Design review of the part built by this model. Coordinates are the model's own, in mm. A direction names the side the tool comes from. Round coordinates to 2 decimals unless told otherwise and drop trailing zeros. Write each loop counter-clockwise with the first axis right and the second up, starting at its lowest first coordinate (ties: lowest second). Pieces come first, ordered by that corner, then holes. Notation, with made-up numbers: (73.25, 5.25) -> (132.25, 5.25) arc R17 ccw to (132.25, 27.25) -> close; hole circle Ø5 at (-10.75, -10). An arc over 180 degrees is marked (long way). One line per question, with ' | ' between items. Start each with the question number.
1) Mouldability with a two-part tool opening along X and no side actions: class faces 5 (the cylindrical face through (-2.17, 13.85, 17.91)), 6 (the cylindrical face through (-13.434, 12.862, 16.727)), 7 (the flat face through (-12, 3, 19)) as +X half, -X half, draft (parallel to the pull), parting line (faces both ways), or undercut.
2) Consider section D-D (y = 3.2). Give the boundary of the cut face in (x, z).
3) Consider section A-A (y = 14.7). Give the boundary of the cut face in (x, z), then the cut area to 3 significant figures.
4) For faces 1 (the flat face through (-3, 6, 19)), 2 (the flat face through (-11, 10, 11.6)), 3 (the flat face through (-9, 21, 17)), 4 (the flat face through (-15, 6, 19)), list the 3-axis set-ups (+Z, -Z, +X, -X, +Y, -Y) from which the entire face can be reached by the end or side of a thin tool; tool diameter is ignored.
5) Consider section B-B (x = -9). Give the boundary of the cut face in (y, z).
6) Consider section C-C (z = 5.25). Give the boundary of the cut face in (x, y), then the cut area to 3 significant figures.
7) Insertion check: pin 1 Ø2 at (x, y) = (-15, 13) entering from -Z; pin 2 Ø9.5 at (x, z) = (-11, 4.5) entering from +Y; pin 3 Ø4 at (x, y) = (-3.25, 3.2) entering from +Z; pin 4 Ø6 at (x, z) = (-12.5, 9) entering from -Y. Each pin has a flat end and moves straight along its axis. Give the tip position at first contact, or say it passes through.
8) For probe 1 along Y at (x, z) = (-14.75, 11.25); probe 2 along Y at (x, z) = (-9, 17.5); probe 3 along Y at (x, z) = (-6.5, 10.75), list the stretches that pass through material, from the lowest coordinate up.
Autodesk Inventor part; units mm, degrees
ref_plane "YZ Plane" through (0, 0, 0) normal (1, 0, 0) x (0, 1, 0)
ref_plane "XZ Plane" through (0, 0, 0) normal (0, 1, 0) x (-1, 0, 0)
ref_plane "XY Plane" through (0, 0, 0) normal (0, 0, 1) x (1, 0, 0)
sketch "Sketch1" plane through (0, 0, 0) normal (0, 0, 1) x (1, 0, 0)
  line L0 (0, 0) -> (-18, 0)
  line L1 (-18, 0) -> (-18, 6)
  line L2 (-18, 6) -> (0, 6)
  line L3 (0, 6) -> (0, 0)
  dimension "d0" = 18
  dimension "d1" = 6
extrude "Extrusion1" add sketch "Sketch1" along normal blind 22
sketch "Sketch2" plane through (0, 0, 22) normal (0, 0, 1) x (1, 0, 0)
  line L0 (-18, 0) -> (0, 0)
  line L1 (0, 0) -> (0, 6)
  line L2 (0, 6) -> (-18, 6)
  line L3 (-18, 6) -> (-18, 0)
  circle A0 centre (-14.75, 3.2) radius 1.25
  circle A1 centre (-3.25, 3.2) radius 1.25
  dimension "d4" = 2.5
  dimension "d5" = 2.5
  dimension "d6" = 2.8
  dimension "d7" = 2.8
  dimension "d8" = 3.25
  dimension "d9" = 3.25
  dimension "d31" = 11.5
extrude "Extrusion2" cut sketch "Sketch2" against normal through all contours A0 | A1
sketch "Sketch3" plane through (0, 0, 0) normal (1, 0, 0) x (0, 0, -1)
  line L0 (0, 6) -> (0, 0)
  line L1 (0, 6) -> (-22, 6)
  line L2 (-22, 0) -> (-22, 6)
  line L3 (0, 0) -> (-22, 0)
  line L4 (0, 6) -> (-22, 6)
  line L5 (-22, 6) -> (-11.6, 6)
  line L6 (-11.6, 6) -> (-11.6, 21)
  line L7 (-11.6, 21) -> (-22, 21)
  line L8 (-22, 21) -> (-22, 6)
  dimension "d12" = 10.4
  dimension "d13" = 15
extrude "Extrusion3" add sketch "Sketch3" against normal up to surface (18 mm away) contours L1 L8 L7 L6
sketch "Sketch4" plane through (0, 6, 11.6) normal (0, 0, -1) x (-1, 0, 0)
  line L0 (18, 0) -> (18, 15)
  line L1 (0, 15) -> (18, 15)
  line L2 (0, 15) -> (0, 0)
  line L3 (18, 0) -> (0, 0)
  circle A0 centre (9, 8.7) radius 4.8
  point P0 (0, -6)
  dimension "d16" = 9.6
  dimension "d17" = 6.3
extrude "Extrusion4" cut sketch "Sketch4" against normal through all contours A0
sketch "Sketch5" plane through (-18, 0, 0) normal (-1, 0, 0) x (0, 0, 1)
  line L0 (22.0213, 0) -> (16.0213, 0)
  line L1 (16.0213, 0) -> (16.0213, 6)
  line L2 (16.0213, 6) -> (22.0213, 6)
  line L3 (22.0213, 6) -> (22.0213, 0)
  point P0 (0, 0)
  dimension "d20" = 6
  dimension "d21" = 6
extrude "Extrusion5" cut sketch "Sketch5" against normal blind 6
sketch "Sketch6" plane through (0, 0, 0) normal (1, 0, 0) x (0, 0, -1)
  line L0 (-22, 6) -> (-22, 0)
  line L1 (-16.0213, 6) -> (-22, 6)
  line L2 (-16.0213, 0) -> (-16.0213, 6)
  line L3 (-22, 0) -> (-16.0213, 0)
  point P0 (0, 0)
extrude "Extrusion6" cut sketch "Sketch6" against normal blind 6
sketch "Sketch7" plane through (0, 0, 0) normal (1, 0, 0) x (0, 0, -1)
  line L0 (-6.6, 12.2) -> (-11.6, 12.2)
  line L1 (-6.6, 17.2) -> (-11.6, 17.2)
  line L2 (-11.6, 21) -> (-11.6, 6)
  line L3 (-22, 6) -> (-22, 21)
  circle A0 centre (-16.8, 14.7) radius 1.4
  point P0 (0, 0)
  dimension "d26" = 2.8
  dimension "d27" = 5.2
  dimension "d28" = 2.5
extrude "Extrusion7" cut sketch "Sketch7" against normal blind 6
equation "\"d9\" = d8"
properties part number "00_micrometer_moun_xystage_china_new"
From the geometry:
1) face 5: draft | face 6: undercut | face 7: -X half
2) outline: (-18, 0) -> (-16, 0) -> (-16, 16.02) -> (-18, 16.02) -> close; (-13.5, 0) -> (-4.5, 0) -> (-4.5, 16.02) -> (-6, 16.02) -> (-6, 22) -> (-12, 22) -> (-12, 16.02) -> (-13.5, 16.02) -> close; (-2, 0) -> (0, 0) -> (0, 16.02) -> (-2, 16.02) -> close
3) outline: (-18, 11.6) -> (-13.8, 11.6) -> (-13.8, 22) -> (-18, 22) -> close; (-4.2, 11.6) -> (0, 11.6) -> (0, 15.4) -> (-4.2, 15.4) -> close; (-4.2, 18.2) -> (0, 18.2) -> (0, 22) -> (-4.2, 22) -> close | area: 75.6 mm2
4) face 1: +Z, +X, -Y | face 2: -Z, +X, -X, +Y | face 3: +Z, -Z, +X, -X, +Y | face 4: +Z, -X, -Y
5) outline: (0, 0) -> (6, 0) -> (6, 11.6) -> (9.9, 11.6) -> (9.9, 22) -> (0, 22) -> close; (19.5, 11.6) -> (21, 11.6) -> (21, 22) -> (19.5, 22) -> close
6) outline: (-18, 0) -> (0, 0) -> (0, 6) -> (-18, 6) -> close; hole circle Ø2.5 at (-14.75, 3.2); hole circle Ø2.5 at (-3.25, 3.2) | area: 98.2 mm2
7) pin 1: stops at z = 11.6 | pin 2: stops at y = 6 | pin 3: stops at z = 16.02 | pin 4: stops at y = 0
8) probe 1: y = 0 to 1.95, 4.45 to 6 | probe 2: y = 0 to 9.9, 19.5 to 21 | probe 3: y = 0 to 6
